from build123d import *

# Parameters (mm, degrees)
SKETCH1_W                = 130
SKETCH1_H                = 190
BOSS_EXTRUDE1_DEPTH      = 6
CUT_EXTRUDE1_REACH       = 117.265
SKETCH2_R                = 10
M8_CLEARANCE_HOLE1_D     = 8.2
M8_CLEARANCE_HOLE1_DEPTH = 19.75
M8_CLEARANCE_HOLE1_TIP   = 2.463528538


with BuildPart() as part:
    # Sketch1 → Boss-Extrude1 (new body)
    with BuildSketch(Plane.XY):
        Rectangle(SKETCH1_W, SKETCH1_H)
    extrude(amount=BOSS_EXTRUDE1_DEPTH)

    # Sketch2 → Cut-Extrude1 (cut, up to next)
    with BuildSketch(Plane.XY.offset(6), mode=Mode.PRIVATE) as cut_extrude1_sk1:
        with Locations((-1.55e-07, 0)):
            Circle(SKETCH2_R)
    cut_extrude1_tool1 = extrude(cut_extrude1_sk1.sketch, amount=-CUT_EXTRUDE1_REACH, mode=Mode.PRIVATE) & part.part
    add(cut_extrude1_tool1.solids().sort_by_distance((0, 0, 6))[0], mode=Mode.SUBTRACT)

    # M8 Clearance Hole1
    with Locations(Plane(origin=(-30, 20, 6), x_dir=(1, 0, 0), z_dir=(0, 0, 1))):
        with Locations((0, 0), (60, 0), (60, -40), (0, -40)):
            Hole(M8_CLEARANCE_HOLE1_D / 2, depth=M8_CLEARANCE_HOLE1_DEPTH)
            with Locations((0, 0, -(M8_CLEARANCE_HOLE1_DEPTH + M8_CLEARANCE_HOLE1_TIP / 2))):  # 118° drill point
                Cone(0, M8_CLEARANCE_HOLE1_D / 2, M8_CLEARANCE_HOLE1_TIP, mode=Mode.SUBTRACT)


solid = part.part
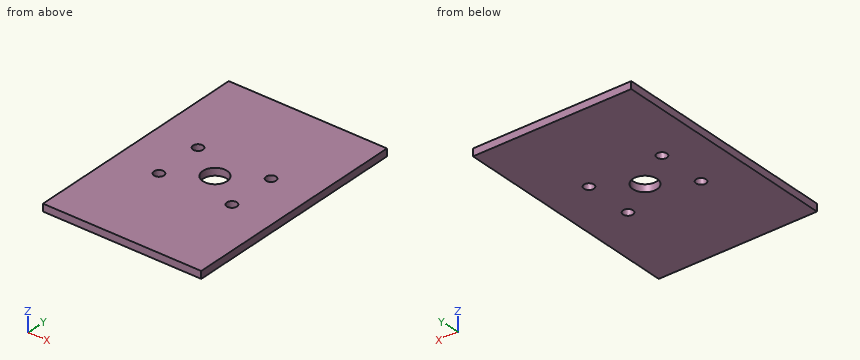
Verification items for the finished model (mm, model axes). Round coordinates to 2 decimals unless told otherwise and drop trailing zeros. Order: outer loops, then holes, each group sorted by start corner. A loop starts at its lowest first (then second) coordinate and runs counter-clockwise, first axis right, second up.
1. Section check B-B on y = -20. Record the cut outline in (x, z).
Final values:
outline: (-65, 0) - (-34.1, 0) - (-34.1, 6) - (-65, 6) - close; (-25.9, 0) - (25.9, 0) - (25.9, 6) - (-25.9, 6) - close; (34.1, 0) - (65, 0) - (65, 6) - (34.1, 6) - close
2. Thickness scan on L1, parallel to Y at x = -30.5, z = 1.05; L2, parallel to Y at x = 0, z = 4.65; L3, parallel to Y at x = 27, z = 2. Record the ranges inside material, lowest first.
Final values:
L1: y = -95 to -24.07, -15.93 to 15.93, 24.07 to 95
L2: y = -95 to -10, 10 to 95
L3: y = -95 to -22.79, -17.21 to 17.21, 22.79 to 95
3. Section check C-C on z = 1.15. Record the cut outline in (x, y).
Final values:
outline: (-65, -95) - (65, -95) - (65, 95) - (-65, 95) - close; hole circle Ø8.2 at (-30, -20); hole circle Ø8.2 at (-30, 20); hole circle Ø20 at (0, 0); hole circle Ø8.2 at (30, -20); hole circle Ø8.2 at (30, 20)
4. Section check A-A on x = -30. Record the cut outline in (y, z), then the cut area to 3 significant figures.
Final values:
outline: (-95, 0) - (-24.1, 0) - (-24.1, 6) - (-95, 6) - close; (-15.9, 0) - (15.9, 0) - (15.9, 6) - (-15.9, 6) - close; (24.1, 0) - (95, 0) - (95, 6) - (24.1, 6) - close
area: 1,040 mm2
5. Section check D-D on x = 0. Record the cut outline in (y, z).
Final values:
outline: (-95, 0) - (-10, 0) - (-10, 6) - (-95, 6) - close; (10, 0) - (95, 0) - (95, 6) - (10, 6) - close
